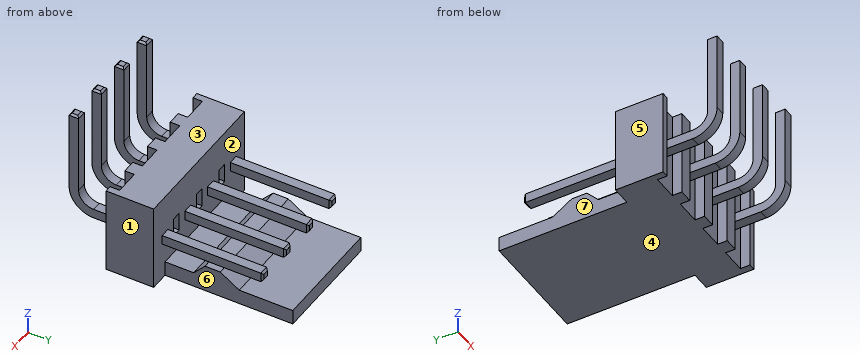
from build123d import *

# Parameters (mm, degrees)
SKETCH1_W            = 8.89
SKETCH1_H            = 5.842
BOSS_EXTRUDE1_DEPTH  = 3.175
BOSS_EXTRUDE2_DEPTH  = 7.62
SKETCH3_W            = 5.842
SKETCH3_H            = 3.175
BOSS_EXTRUDE3_DEPTH  = 1.27
SKETCH4_W            = 1.651
SKETCH4_H            = 0.635
CUT_EXTRUDE1_DEPTH   = 13.735698656
SKETCH5_W            = 0.635
SKETCH5_H            = 0.635
BOSS_EXTRUDE4_DEPTH  = 3.6725
SKETCH6_W            = 0.635
SKETCH6_H            = 0.635
BOSS_EXTRUDE5_DEPTH  = 6.4543
SKETCH7_W            = 1.651
SKETCH7_H            = 0.635
CUT_EXTRUDE2_DEPTH   = 15.867320547
SKETCH8_W            = 0.635
SKETCH8_H            = 0.635
BOSS_EXTRUDE6_DEPTH  = 3.6725
SKETCH9_W            = 0.635
SKETCH9_H            = 0.635
BOSS_EXTRUDE7_DEPTH  = 6.4543
SKETCH10_W           = 1.651
SKETCH10_H           = 0.635
CUT_EXTRUDE3_DEPTH   = 15.867320547
SKETCH11_W           = 0.635
SKETCH11_H           = 0.635
BOSS_EXTRUDE8_DEPTH  = 3.6725
SKETCH12_W           = 0.635
SKETCH12_H           = 0.635
BOSS_EXTRUDE9_DEPTH  = 6.4543
SKETCH13_W           = 1.651
SKETCH13_H           = 0.635
CUT_EXTRUDE4_DEPTH   = 15.867320547
SKETCH14_W           = 0.635
SKETCH14_H           = 0.635
BOSS_EXTRUDE10_DEPTH = 3.6725
SKETCH15_W           = 0.635
SKETCH15_H           = 0.635
BOSS_EXTRUDE11_DEPTH = 6.4543
SKETCH16_W           = 0.635
SKETCH16_H           = 0.635
BOSS_EXTRUDE12_DEPTH = 6.71
SKETCH17_W           = 0.635
SKETCH17_H           = 0.635
BOSS_EXTRUDE13_DEPTH = 6.71
SKETCH18_W           = 0.635
SKETCH18_H           = 0.635
BOSS_EXTRUDE14_DEPTH = 6.71
SKETCH19_W           = 0.635
SKETCH19_H           = 0.635
BOSS_EXTRUDE15_DEPTH = 6.71
SKETCH20_W           = 0.635
SKETCH20_H           = 1.27
CUT_EXTRUDE5_DEPTH   = 1.27
SKETCH21_W           = 0.635
SKETCH21_H           = 1.27
CUT_EXTRUDE6_DEPTH   = 1.27
SKETCH22_W           = 0.635
SKETCH22_H           = 1.27
CUT_EXTRUDE7_DEPTH   = 1.27
CHAMFER1_SIZE        = 0.127
CHAMFER2_SIZE        = 0.753913762
CHAMFER2_SIZE2       = 0.55706549
FILLET1_R            = 1
FILLET2_R            = 1.635


with BuildPart() as part:
    # Sketch1 → Boss-Extrude1 (new body)
    with BuildSketch(Plane.XZ.offset(1.5875)):
        with Locations((-0.635, 0.0508)):
            Rectangle(SKETCH1_W, SKETCH1_H)
    extrude(amount=-BOSS_EXTRUDE1_DEPTH)

    # Sketch2 → Boss-Extrude2 (add)
    with BuildSketch(Plane(origin=(3.81, 0, 0), x_dir=(0, 0, -1), z_dir=(1, 0, 0))):
        Polygon((0.651, 4.6355), (1.8702, 3.4925), (1.8702, 1.5875), (2.8702, 1.5875), (2.8702, 10.1125), (1.8702, 10.1125), (1.8702, 6.5405), align=None)
    extrude(amount=-BOSS_EXTRUDE2_DEPTH)

    # Sketch3 → Boss-Extrude3 (add)
    with BuildSketch(Plane(origin=(3.81, 0, 0), x_dir=(0, 0, -1), z_dir=(1, 0, 0))):
        with Locations((-0.0508, 0)):
            Rectangle(SKETCH3_W, SKETCH3_H)
    extrude(amount=BOSS_EXTRUDE3_DEPTH)

    # Sketch4 → Cut-Extrude1 (cut, through all)
    with BuildSketch(Plane(origin=(0, 0, -2.8702), x_dir=(-1, 0, 0), z_dir=(0, 0, -1))):
        with Locations((1.27, -1.27)):
            Rectangle(SKETCH4_W, SKETCH4_H)
    extrude(amount=-CUT_EXTRUDE1_DEPTH, mode=Mode.SUBTRACT)

    # Sketch5 → Boss-Extrude4 (add)
    with BuildSketch(Plane.XZ.offset(0.9525)):
        with Locations((-1.27, 0)):
            Rectangle(SKETCH5_W, SKETCH5_H)
    extrude(amount=BOSS_EXTRUDE4_DEPTH)

    # Sketch6 → Boss-Extrude5 (add)
    with BuildSketch(Plane.XY.offset(0.3175)):
        with Locations((-1.27, -4.3075)):
            Rectangle(SKETCH6_W, SKETCH6_H)
    extrude(amount=BOSS_EXTRUDE5_DEPTH)

    # Sketch7 → Cut-Extrude2 (cut, through all)
    with BuildSketch(Plane(origin=(0, 0, -2.8702), x_dir=(-1, 0, 0), z_dir=(0, 0, -1))):
        with Locations((-1.27, -1.27)):
            Rectangle(SKETCH7_W, SKETCH7_H)
    extrude(amount=-CUT_EXTRUDE2_DEPTH, mode=Mode.SUBTRACT)

    # Sketch8 → Boss-Extrude6 (add)
    with BuildSketch(Plane.XZ.offset(0.9525)):
        with Locations((1.27, 0)):
            Rectangle(SKETCH8_W, SKETCH8_H)
    extrude(amount=BOSS_EXTRUDE6_DEPTH)

    # Sketch9 → Boss-Extrude7 (add)
    with BuildSketch(Plane.XY.offset(0.3175)):
        with Locations((1.27, -4.3075)):
            Rectangle(SKETCH9_W, SKETCH9_H)
    extrude(amount=BOSS_EXTRUDE7_DEPTH)

    # Sketch10 → Cut-Extrude3 (cut, through all)
    with BuildSketch(Plane(origin=(0, 0, -2.8702), x_dir=(-1, 0, 0), z_dir=(0, 0, -1))):
        with Locations((3.81, -1.27)):
            Rectangle(SKETCH10_W, SKETCH10_H)
    extrude(amount=-CUT_EXTRUDE3_DEPTH, mode=Mode.SUBTRACT)

    # Sketch11 → Boss-Extrude8 (add)
    with BuildSketch(Plane.XZ.offset(0.9525)):
        with Locations((-3.81, 0)):
            Rectangle(SKETCH11_W, SKETCH11_H)
    extrude(amount=BOSS_EXTRUDE8_DEPTH)

    # Sketch12 → Boss-Extrude9 (add)
    with BuildSketch(Plane.XY.offset(0.3175)):
        with Locations((-3.81, -4.3075)):
            Rectangle(SKETCH12_W, SKETCH12_H)
    extrude(amount=BOSS_EXTRUDE9_DEPTH)

    # Sketch13 → Cut-Extrude4 (cut, through all)
    with BuildSketch(Plane(origin=(0, 0, -2.8702), x_dir=(-1, 0, 0), z_dir=(0, 0, -1))):
        with Locations((-3.81, -1.27)):
            Rectangle(SKETCH13_W, SKETCH13_H)
    extrude(amount=-CUT_EXTRUDE4_DEPTH, mode=Mode.SUBTRACT)

    # Sketch14 → Boss-Extrude10 (add)
    with BuildSketch(Plane.XZ.offset(0.9525)):
        with Locations((3.81, 0)):
            Rectangle(SKETCH14_W, SKETCH14_H)
    extrude(amount=BOSS_EXTRUDE10_DEPTH)

    # Sketch15 → Boss-Extrude11 (add)
    with BuildSketch(Plane.XY.offset(0.3175)):
        with Locations((3.81, -4.3075)):
            Rectangle(SKETCH15_W, SKETCH15_H)
    extrude(amount=BOSS_EXTRUDE11_DEPTH)

    # Sketch16 → Boss-Extrude12 (add)
    with BuildSketch(Plane(origin=(0, 1.5875, 0), x_dir=(-1, 0, 0), z_dir=(0, 1, 0))):
        with Locations((-3.81, 0)):
            Rectangle(SKETCH16_W, SKETCH16_H)
    extrude(amount=BOSS_EXTRUDE12_DEPTH)

    # Sketch17 → Boss-Extrude13 (add)
    with BuildSketch(Plane(origin=(0, 1.5875, 0), x_dir=(-1, 0, 0), z_dir=(0, 1, 0))):
        with Locations((-1.27, 0)):
            Rectangle(SKETCH17_W, SKETCH17_H)
    extrude(amount=BOSS_EXTRUDE13_DEPTH)

    # Sketch18 → Boss-Extrude14 (add)
    with BuildSketch(Plane(origin=(0, 1.5875, 0), x_dir=(-1, 0, 0), z_dir=(0, 1, 0))):
        with Locations((1.27, 0)):
            Rectangle(SKETCH18_W, SKETCH18_H)
    extrude(amount=BOSS_EXTRUDE14_DEPTH)

    # Sketch19 → Boss-Extrude15 (add)
    with BuildSketch(Plane(origin=(0, 1.5875, 0), x_dir=(-1, 0, 0), z_dir=(0, 1, 0))):
        with Locations((3.81, 0)):
            Rectangle(SKETCH19_W, SKETCH19_H)
    extrude(amount=BOSS_EXTRUDE15_DEPTH)

    # Sketch20 → Cut-Extrude5 (cut)
    with BuildSketch(Plane(origin=(0, 1.5875, 0), x_dir=(-1, 0, 0), z_dir=(0, 1, 0))):
        with Locations((-2.54, 0)):
            Rectangle(SKETCH20_W, SKETCH20_H)
    extrude(amount=-CUT_EXTRUDE5_DEPTH, mode=Mode.SUBTRACT)

    # Sketch21 → Cut-Extrude6 (cut)
    with BuildSketch(Plane(origin=(0, 1.5875, 0), x_dir=(-1, 0, 0), z_dir=(0, 1, 0))):
        Rectangle(SKETCH21_W, SKETCH21_H)
    extrude(amount=-CUT_EXTRUDE6_DEPTH, mode=Mode.SUBTRACT)

    # Sketch22 → Cut-Extrude7 (cut)
    with BuildSketch(Plane(origin=(0, 1.5875, 0), x_dir=(-1, 0, 0), z_dir=(0, 1, 0))):
        with Locations((2.54, 0)):
            Rectangle(SKETCH22_W, SKETCH22_H)
    extrude(amount=-CUT_EXTRUDE7_DEPTH, mode=Mode.SUBTRACT)

    # Chamfer1
    chamfer1_edges = [part.edges().sort_by_distance(p)[0] for p in [
        (1.5875, -4.3075, 6.7718),
        (1.27, -3.99, 6.7718),
        (0.9525, -4.3075, 6.7718),
        (1.27, -4.625, 6.7718),
        (-3.4925, -4.3075, 6.7718),
        (-3.81, -3.99, 6.7718),
        (-4.1275, -4.3075, 6.7718),
        (-3.81, -4.625, 6.7718),
        (4.1275, -4.3075, 6.7718),
        (3.81, -3.99, 6.7718),
        (3.4925, -4.3075, 6.7718),
        (3.81, -4.625, 6.7718),
        (4.1275, 8.2975, 0),
        (3.81, 8.2975, -0.3175),
        (3.4925, 8.2975, 0),
        (3.81, 8.2975, 0.3175),
        (0.9525, 8.2975, 0),
        (1.27, 8.2975, 0.3175),
        (1.5875, 8.2975, 0),
        (1.27, 8.2975, -0.3175),
        (-0.9525, 8.2975, 0),
        (-1.27, 8.2975, -0.3175),
        (-1.5875, 8.2975, 0),
        (-1.27, 8.2975, 0.3175),
        (-3.81, 8.2975, -0.3175),
        (-4.1275, 8.2975, 0),
        (-3.81, 8.2975, 0.3175),
        (-3.4925, 8.2975, 0),
        (-1.27, -3.99, 6.7718),
        (-1.5875, -4.3075, 6.7718),
        (-1.27, -4.625, 6.7718),
        (-0.9525, -4.3075, 6.7718),
    ]]
    chamfer(chamfer1_edges, length=CHAMFER1_SIZE)

    # Chamfer2
    chamfer2_edges = [part.edges().sort_by_distance(p)[0] for p in [
        (0, 4.6355, -0.651),
    ]]
    chamfer2_side = [part.faces().sort_by_distance(p)[0] for p in [
        (0, 5.588, -1.2606),
    ]]
    chamfer(chamfer2_edges, length=CHAMFER2_SIZE, length2=CHAMFER2_SIZE2, reference=chamfer2_side[0])

    # Fillet1
    fillet1_edges = [part.edges().sort_by_distance(p)[0] for p in [
        (1.27, -3.99, 0.3175),
        (-3.81, -3.99, 0.3175),
        (3.81, -3.99, 0.3175),
        (-1.27, -3.99, 0.3175),
    ]]
    fillet(fillet1_edges, radius=FILLET1_R)

    # Fillet2
    fillet2_edges = [part.edges().sort_by_distance(p)[0] for p in [
        (1.27, -4.625, -0.3175),
        (-3.81, -4.625, -0.3175),
        (3.81, -4.625, -0.3175),
        (-1.27, -4.625, -0.3175),
    ]]
    fillet(fillet2_edges, radius=FILLET2_R)


solid = part.part
Check sheet for the modelled part. Datum: model origin and axes. Units: mm. Face numbers are marked on the shaded views. A direction names the side the tool comes from. Coordinates: 2 decimals unless noted, no trailing zeros. Loops run counter-clockwise (first coordinate to the right, second up) from the corner with the lowest first, then second, coordinate; pieces in that order, holes last. Notation, with made-up numbers: (-22, -16) -> (-4, -16) arc R29 cw to (-4, 6) -> close; hole circle Ø4 at (86.5, 18). An arc over 180 degrees is marked (long way). Answer in a Markdown table with one row per item.
1. Release check for a two-part mould opening along Y. For the marked faces 1 and 2 record: released by +Y, released by -Y, zero draft, split by the parting line, or undercut.
Check values:
| item | result |
|---|---|
| face 1 | zero draft |
| face 2 | undercut |
2. Sectioned sample at A-A, the plane y = 3.25. Record the boundary of the cut face in (x, z).
Check values:
| item | result |
|---|---|
| outline | (-4.13, -0.32) -> (-3.49, -0.32) -> (-3.49, 0.32) -> (-4.13, 0.32) -> close; (-3.81, -2.87) -> (3.81, -2.87) -> (3.81, -1.87) -> (-3.81, -1.87) -> close; (-1.59, -0.32) -> (-0.95, -0.32) -> (-0.95, 0.32) -> (-1.59, 0.32) -> close; (0.95, -0.32) -> (1.59, -0.32) -> (1.59, 0.32) -> (0.95, 0.32) -> close; (3.49, -0.32) -> (4.13, -0.32) -> (4.13, 0.32) -> (3.49, 0.32) -> close |
3. Sectioned sample at B-B, the plane y = 1.25. Record the boundary of the cut face in (x, z) (1 decimal).
Check values:
| item | result |
|---|---|
| outline | (-5.1, -2.9) -> (5.1, -2.9) -> (5.1, 3) -> (-5.1, 3) -> close; hole (-2.9, -0.6) -> (-2.2, -0.6) -> (-2.2, 0.6) -> (-2.9, 0.6) -> close; hole (-0.3, -0.6) -> (0.3, -0.6) -> (0.3, 0.6) -> (-0.3, 0.6) -> close; hole (2.2, -0.6) -> (2.9, -0.6) -> (2.9, 0.6) -> (2.2, 0.6) -> close |
4. Go/stop test with flat-tipped pins: pin 1 (3 mm diameter, centred on y = 3.5, z = 3.5, fed in from +X); pin 2 (2 mm diameter, centred on y = 4.5, z = -2.5, fed in from -X); pin 3 (0.5 mm diameter, centred on x = 1, y = 5, fed in from +Z); pin 4 (0.7 mm diameter, centred on x = 2.5, y = 1, fed in from +Z). Record where each tip stops, or that it passes through.
Check values:
| item | result |
|---|---|
| pin 1 | passes through |
| pin 2 | stops at x = -3.81 |
| pin 3 | stops at z = 0.32 |
| pin 4 | stops at z = 2.97 |
5. Sectioned sample at C-C, the plane x = -2.5. Record the boundary of the cut face in (y, z) (1 decimal).
Check values:
| item | result |
|---|---|
| outline | (-1.6, -2.9) -> (10.1, -2.9) -> (10.1, -1.9) -> (6.5, -1.9) -> (5.3, -1.1) -> (4.3, -1.1) -> (3.5, -1.9) -> (1.6, -1.9) -> (1.6, -0.6) -> (0.3, -0.6) -> (0.3, 0.6) -> (1.6, 0.6) -> (1.6, 3) -> (-1.6, 3) -> close |
6. Material ranges on line 1 along Z through (x, y) = (1, 4.5); line 2 along Z through (x, y) = (0.25, 1.5) (3 decimals); line 3 along Y through (x, z) = (1, 2.5) (1 decimal), recorded low to high. Write a range as [from, to].
Check values:
| item | result |
|---|---|
| line 1 | z = [-2.87, -1.06], [-0.32, 0.32] |
| line 2 | z = [-2.87, -0.635], [0.635, 2.972] |
| line 3 | y = [-4.6, -4], [-1, 1.6] |
7. Access from +Z, -Z, +X, -X, +Y, -Y to the whole of each face (thin tool, end or side, straight path). Record for the marked faces 3, 4, 5, 6 and 7.
Check values:
| item | result |
|---|---|
| face 3 | +Z, +X, -X, +Y |
| face 4 | -Z, +X, -X, +Y, -Y |
| face 5 | +Z, -Z, -X, +Y, -Y |
| face 6 | -Z, +X, +Y |
| face 7 | -Z, -X, +Y |
